Check sheet for the modelled part. Datum: model origin and axes. Units: mm. Face numbers are marked on the shaded views. Coordinates: 2 decimals unless noted, no trailing zeros. Write each loop counter-clockwise with the first axis right and the second up, starting at its lowest first coordinate (ties: lowest second). Pieces come first, ordered by that corner, then holes. Notation, with made-up numbers: M 62,50.25 L 68,50.25 A25 cw 68,86.25 Z; hole C -17.75,-1.75 d3. An arc over 180 degrees is marked long. Answer as CSV lines item,"result".
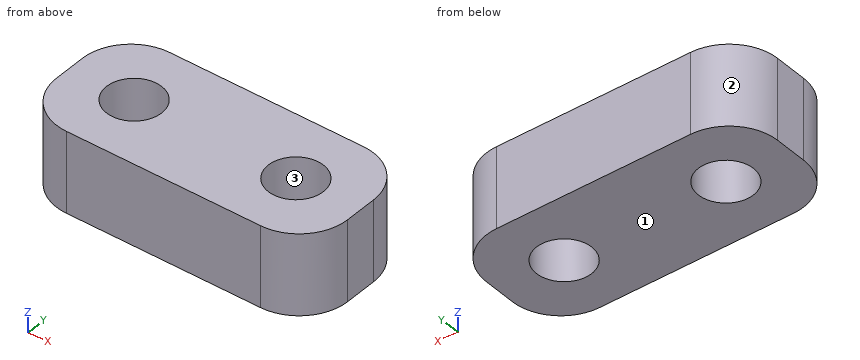
from build123d import *

# Parameters (mm, degrees)
SKETCH1_W            = 18
SKETCH1_H            = 8
BOSS_EXTRUDE1_DEPTH  = 2.5
M3_CLEARANCE_HOLE1_D = 3.4
FILLET1_R            = 3


with BuildPart() as part:
    # Sketch1 → Boss-Extrude1 (new body, symmetric)
    with BuildSketch(Plane.XY):
        Rectangle(SKETCH1_W, SKETCH1_H)
    extrude(amount=BOSS_EXTRUDE1_DEPTH, both=True)

    # M3 Clearance Hole1 (through all)
    with Locations(Plane.XY.offset(2.5)):
        with Locations((-5, 0), (5, 0)):
            Hole(M3_CLEARANCE_HOLE1_D / 2)

    # Fillet1
    fillet1_edges = [part.edges().sort_by_distance(p)[0] for p in [
        (9, -4, 0),
        (-9, -4, 0),
        (-9, 4, 0),
        (9, 4, 0),
    ]]
    fillet(fillet1_edges, radius=FILLET1_R)


solid = part.part
1) Mould release check, pull along X, two halves, no side actions. Record for the marked faces 1, 2 and 3: pulls with the +X half, pulls with the -X half, needs draft (parallel to the pull), parting line crosses it, or undercut.
Answer key:
face 1,"needs draft"
face 2,"pulls with the -X half"
face 3,"undercut"
2) Section check B-B, the plane z = -1.2. Record the boundary of the cut face in (x, y).
Answer key:
outline,"M -9,-1 A3 ccw -6,-4 L 6,-4 A3 ccw 9,-1 L 9,1 A3 ccw 6,4 L -6,4 A3 ccw -9,1 Z; hole C -5,0 d3.4; hole C 5,0 d3.4"
3) Depth check by flat-ended pin: P1, Ø3, axis at x = -5, y = 0, coming from the +Z side. Enter the tip coordinate at first touch or a pass-through.
Answer key:
P1,"passes through"
4) Section check A-A, the plane y = 0. Record the boundary of the cut face in (x, z).
Answer key:
outline,"M -9,-2.5 L -6.7,-2.5 L -6.7,2.5 L -9,2.5 Z; M -3.3,-2.5 L 3.3,-2.5 L 3.3,2.5 L -3.3,2.5 Z; M 6.7,-2.5 L 9,-2.5 L 9,2.5 L 6.7,2.5 Z"
5) Section check D-D, the plane y = 1.5. Record the boundary of the cut face in (x, z), plus the area to 3 significant figures.
Answer key:
outline,"M -8.96,-2.5 L -5.8,-2.5 L -5.8,2.5 L -8.96,2.5 Z; M -4.2,-2.5 L 4.2,-2.5 L 4.2,2.5 L -4.2,2.5 Z; M 5.8,-2.5 L 8.96,-2.5 L 8.96,2.5 L 5.8,2.5 Z"
area,"73.6 mm2"
6) Thickness scan on line 1 along Y through (x, z) = (-5, -0.1); line 2 along X through (y, z) = (-0.25, -0.85); line 3 along Y through (x, z) = (6.5, -0.35). Record the ranges inside material, lowest first.
Answer key:
line 1,"y = -4 to -1.7, 1.7 to 4"
line 2,"x = -9 to -6.68, -3.32 to 3.32, 6.68 to 9"
line 3,"y = -3.96 to -0.8, 0.8 to 3.96"
7) Section check C-C, the plane x = -5. Record the boundary of the cut face in (y, z), plus the area to 3 significant figures.
Answer key:
outline,"M -4,-2.5 L -1.7,-2.5 L -1.7,2.5 L -4,2.5 Z; M 1.7,-2.5 L 4,-2.5 L 4,2.5 L 1.7,2.5 Z"
area,"23.0 mm2"
